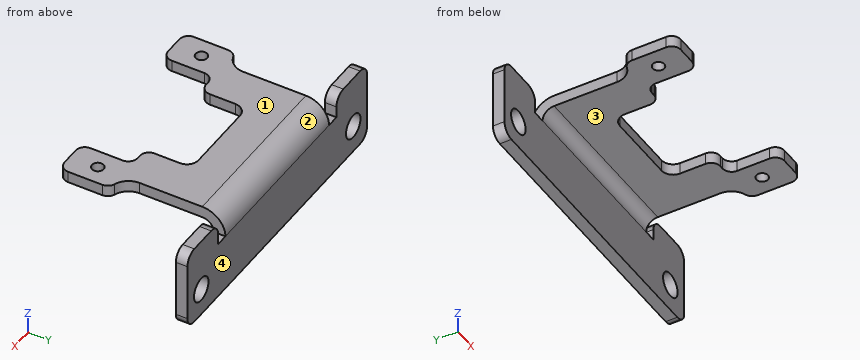
```python
from build123d import *

# Parameters (mm, degrees)
ESQUISSE1_R                           = 2.5
T_LE_DE_BASE_PLI_E1_DEPTH             = 5
T_LE_PLI_E_SUR_AR_TE1_STRIP_W         = 30
T_LE_PLI_E_SUR_AR_TE1_STRIP_H         = 5
T_LE_PLI_E_SUR_AR_TE1_STRIP_CUT_DEPTH = 130
T_LE_PLI_E_SUR_AR_TE1_DEPTH           = 130
CONG_1_R                              = 5
ESQUISSE7_R                           = 5.25
EXTRUSION2_DEPTH                      = 10
ESQUISSE8_W                           = 27.5
ESQUISSE8_H                           = 20
EXTRUSION3_DEPTH                      = 10
PATTE1_DEPTH                          = 5


# Sheet-metal steps are written as plain solids
with BuildPart() as part:
    # Esquisse1 → Tôle de base pliée1 (new body)
    with BuildSketch(Plane.XY):
        with BuildLine():
            Line((29.5, 6), (29.5, -8))
            ThreePointArc((29.5, -8), (30.671572875, -10.828427125), (33.5, -12))
            Line((33.5, -12), (41.5, -12))
            ThreePointArc((41.5, -12), (44.328427125, -10.828427125), (45.5, -8))
            Line((45.5, -8), (45.5, 6.686291501))
            ThreePointArc((45.5, 6.686291501), (44.765986324, 8.995692578), (42.833333333, 10.457527667))
            ThreePointArc((42.833333333, 10.457527667), (38.968027353, 13.381197846), (37.5, 18))
            Line((37.5, 18), (37.5, 35))
            ThreePointArc((37.5, 35), (40.428932188, 42.071067812), (47.5, 45))
            Line((47.5, 45), (65, 45))
            Line((65, 45), (65, 50))
            Line((65, 50), (-65, 50))
            Line((-65, 50), (-65, 45))
            Line((-65, 45), (-47.5, 45))
            ThreePointArc((-47.5, 45), (-40.428932188, 42.071067812), (-37.5, 35))
            Line((-37.5, 35), (-37.5, 18))
            ThreePointArc((-37.5, 18), (-38.968027353, 13.381197846), (-42.833333333, 10.457527667))
            ThreePointArc((-42.833333333, 10.457527667), (-44.765986324, 8.995692578), (-45.5, 6.686291501))
            Line((-45.5, 6.686291501), (-45.5, -8))
            ThreePointArc((-45.5, -8), (-44.328427125, -10.828427125), (-41.5, -12))
            Line((-41.5, -12), (-33.5, -12))
            ThreePointArc((-33.5, -12), (-30.671572875, -10.828427125), (-29.5, -8))
            Line((-29.5, -8), (-29.5, 6))
            ThreePointArc((-29.5, 6), (-28.328427125, 8.828427125), (-25.5, 10))
            Line((-25.5, 10), (-24, 10))
            ThreePointArc((-24, 10), (-21.171572875, 11.171572875), (-20, 14))
            Line((-20, 14), (-20, 25))
            ThreePointArc((-20, 25), (-18.535533906, 28.535533906), (-15, 30))
            Line((-15, 30), (15, 30))
            ThreePointArc((15, 30), (18.535533906, 28.535533906), (20, 25))
            Line((20, 25), (20, 14))
            ThreePointArc((20, 14), (21.171572875, 11.171572875), (24, 10))
            Line((24, 10), (25.5, 10))
            ThreePointArc((25.5, 10), (28.328427125, 8.828427125), (29.5, 6))
        make_face()
        with Locations((37.5, 0)):
            Circle(ESQUISSE1_R, mode=Mode.SUBTRACT)
        with Locations(Location((-37.5, 0, 0), (0, 0, 180))):
            Circle(ESQUISSE1_R, mode=Mode.SUBTRACT)
    extrude(amount=T_LE_DE_BASE_PLI_E1_DEPTH)

    # Tôle pliée sur arête1 strip (across the edge) → Tôle pliée sur arête1 strip cut (cut)
    with BuildSketch(Plane(origin=(-65, 50, 0), x_dir=(0, -1, 0), z_dir=(1, 0, 0))):
        with Locations((-10, -2.5)):
            Rectangle(T_LE_PLI_E_SUR_AR_TE1_STRIP_W, T_LE_PLI_E_SUR_AR_TE1_STRIP_H)
    extrude(amount=T_LE_PLI_E_SUR_AR_TE1_STRIP_CUT_DEPTH, mode=Mode.SUBTRACT)

    # Tôle pliée sur arête1 section (across the edge) → Tôle pliée sur arête1 (add)
    with BuildSketch(Plane(origin=(-65, 50, 0), x_dir=(0, -1, 0), z_dir=(1, 0, 0))):
        with BuildLine():
            Line((-5, 5), (-5, 30))
            Line((-5, 30), (0, 30))
            Line((0, 30), (0, 5))
            ThreePointArc((0, 5), (1.464466094, 1.464466094), (5, 0))
            Line((5, 0), (5, -5))
            ThreePointArc((5, -5), (-2.071067812, -2.071067812), (-5, 5))
        make_face()
    extrude(amount=T_LE_PLI_E_SUR_AR_TE1_DEPTH)

    # Congé1
    cong_1_edges = [part.edges().sort_by_distance(p)[0] for p in [
        (-65, 45, 2.5),
        (65, 45, 2.5),
        (-65, 52.5, -30),
        (65, 52.5, -30),
    ]]
    fillet(cong_1_edges, radius=CONG_1_R - 0.0001)  # a hair under: the kernel refuses the full size

    # Esquisse7 → Extrusion2 (cut)
    with BuildSketch(Plane(origin=(0, 55, 0), x_dir=(1, 0, 0), z_dir=(0, 1, 0))):
        with Locations(Location((55, 18, 0), (0, 0, 270))):
            Circle(ESQUISSE7_R)
        with Locations(Location((-55, 18, 0), (0, 0, 90))):
            Circle(ESQUISSE7_R)
    extrude(amount=-EXTRUSION2_DEPTH, mode=Mode.SUBTRACT)

    # Esquisse8 → Extrusion3 (cut)
    with BuildSketch(Plane.XY.offset(5)):
        with Locations((51.25, 45)):
            Rectangle(ESQUISSE8_W, ESQUISSE8_H)
        with Locations((-51.25, 45)):
            Rectangle(ESQUISSE8_W, ESQUISSE8_H)
    extrude(amount=-EXTRUSION3_DEPTH, mode=Mode.SUBTRACT)

    # Esquisse9 → Patte1 (add)
    with BuildSketch(Plane(origin=(0, 55, 0), x_dir=(1, 0, 0), z_dir=(0, 1, 0))):
        with BuildLine():
            Line((-65, 5), (-42.833333333, 5))
            Line((-42.833333333, 5), (-42.833333333, 0))
            ThreePointArc((-42.833333333, 0), (-44.297799427, -3.535533906), (-47.833333333, -5))
            Line((-47.833333333, -5), (-60, -5))
            ThreePointArc((-60, -5), (-63.535533906, -3.535533906), (-65, 0))
            Line((-65, 0), (-65, 5))
        make_face()
        with BuildLine():
            Line((65, 5), (42.833333333, 5))
            Line((42.833333333, 5), (42.833333333, 0))
            ThreePointArc((42.833333333, 0), (44.297799427, -3.535533906), (47.833333333, -5))
            Line((47.833333333, -5), (60, -5))
            ThreePointArc((60, -5), (63.535533906, -3.535533906), (65, 0))
            Line((65, 0), (65, 5))
        make_face()
    extrude(amount=-PATTE1_DEPTH)


solid = part.part
```
Check sheet for the modelled part. Datum: model origin and axes. Units: mm. Face numbers are marked on the shaded views. A direction names the side the tool comes from. Round coordinates to 2 decimals unless told otherwise and drop trailing zeros. Order: outer loops, then holes, each group sorted by start corner. A loop starts at its lowest first (then second) coordinate and runs counter-clockwise, first axis right, second up. Notation, with made-up numbers: (-23, 20) -> (-14, 20) arc R21 cw to (-14, 28) -> close; hole circle Ø8 at (75.5, -34). An arc over 180 degrees is marked (long way). One line per item, written item: value. Start each with the question number.
Q1. Set-up check for the marked faces 3 and 4: record each of +Z, -Z, +X, -X, +Y, -Y from which the full face is reachable in a straight line by a thin tool's end or side.
Q2. Gauge pin test, flat ends, axial feed: pin 1 Ø4.5 at (x, y) = (37.5, 0) entering from +Z; pin 2 Ø2.5 at (x, y) = (-40, 52) entering from +Z; pin 3 Ø1.5 at (x, y) = (-3.5, 40.5) entering from -Z; pin 4 Ø0.8 at (x, z) = (-25, 3) entering from -Y. Record the tip position at first contact, or that the pin passes through.
Q3. Mould release check, pull along X, two halves, no side actions. Record for the marked faces 1 and 2: pulls with the +X half, pulls with the -X half, needs draft (parallel to the pull), parting line crosses it, or undercut.
Q4. Cross-section at B-B (y = 0). Record the boundary of the cut face in (x, z), and give its area (3 significant figures).
Q5. Cross-section at D-D (z = 1.5). Give the number of separate pieces and of enclosed holes in the cut face, and give its area (3 significant figures).
Q6. Cross-section at C-C (x = -55). Record the boundary of the cut face in (y, z).
Q7. Thickness scan on line 1 (X direction, y = 51.3, z = -18); line 2 (Y direction, x = 17, z = -26); line 3 (Z direction, x = -55, y = 52.8). Record the ranges inside material, lowest first.
Q8. Cross-section at A-A (z = -18). Record the boundary of the cut face in (x, y).
Completed:
1. face 3: -Z, +X, -X, -Y
1. face 4: +Z, -Z, +X, -X, +Y
2. pin 1: passes through
2. pin 2: stops at z = -5
2. pin 3: stops at z = 0
2. pin 4: stops at y = 10
3. face 1: needs draft
3. face 2: undercut
4. outline: (-45.5, 0) -> (-40, 0) -> (-40, 5) -> (-45.5, 5) -> close; (-35, 0) -> (-29.5, 0) -> (-29.5, 5) -> (-35, 5) -> close; (29.5, 0) -> (35, 0) -> (35, 5) -> (29.5, 5) -> close; (40, 0) -> (45.5, 0) -> (45.5, 5) -> (40, 5) -> close
4. area: 110 mm²
5. separate pieces: 3
5. enclosed holes: 2
5. area: 3,300 mm²
6. outline: (50, -30) -> (55, -30) -> (55, -23.25) -> (50, -23.25) -> close; (50, -12.75) -> (55, -12.75) -> (55, 5) -> (50, 5) -> close
7. line 1: x = -65 to -60.25, -49.75 to 49.75, 60.25 to 65
7. line 2: y = 50 to 55
7. line 3: z = -30 to -23.25, -12.75 to 5
8. outline: (-65, 50) -> (-60.25, 50) -> (-60.25, 55) -> (-65, 55) -> close; (-49.75, 50) -> (49.75, 50) -> (49.75, 55) -> (-49.75, 55) -> close; (60.25, 50) -> (65, 50) -> (65, 55) -> (60.25, 55) -> close
